Build history of the part. All positions in model axes, mm. Coordinates: 2 decimals unless noted, no trailing zeros. Loops run counter-clockwise (first coordinate to the right, second up) from the corner with the lowest first, then second, coordinate; pieces in that order, holes last. Notation, with made-up numbers: (-0.75, 59.25) - (33.25, 59.25) arc R25 ccw to (33.25, 88.25) - close; hole circle Ø10 at (59, -22). An arc over 180 degrees is marked (long way). One line per item, written item: value.
```python
from build123d import *

# Parameters (mm, degrees)
BOSS_EXTRUDE1_DEPTH                          = 2.5
CSK_FOR_M2_5_COUNTERSUNK_FLAT_HEAD_S_2_COUNT = 2
CSK_FOR_M2_5_COUNTERSUNK_FLAT_HEAD_S_2_PITCH = 24
CSK_FOR_M2_5_COUNTERSUNK_FLAT_HEAD_S_3_COUNT = 2
CSK_FOR_M2_5_COUNTERSUNK_FLAT_HEAD_S_3_PITCH = 114
CSK_FOR_M2_5_COUNTERSUNK_FLAT_HEAD_S_4_COUNT = 2
CSK_FOR_M2_5_COUNTERSUNK_FLAT_HEAD_S_4_PITCH = 116.498927034
SKETCH4_R                                    = 10.25
CUT_EXTRUDE1_DEPTH                           = 132.231695022


with BuildPart() as part:
    # Sketch1 → Boss-Extrude1 (new body)
    with BuildSketch(Plane.XY):
        with BuildLine():
            Line((-63.122572744, 90.432106023), (-63.122572744, -25.567893977))
            ThreePointArc((-63.122572744, -25.567893977), (-63.708359182, -26.98210754), (-65.122572744, -27.567893977))
            Line((-65.122572744, -27.567893977), (-91.122572744, -27.567893977))
            ThreePointArc((-91.122572744, -27.567893977), (-92.536786306, -26.98210754), (-93.122572744, -25.567893977))
            Line((-93.122572744, -25.567893977), (-93.122572744, 90.432106023))
            ThreePointArc((-93.122572744, 90.432106023), (-92.536786306, 91.846319585), (-91.122572744, 92.432106023))
            Line((-91.122572744, 92.432106023), (-65.122572744, 92.432106023))
            ThreePointArc((-65.122572744, 92.432106023), (-63.708359182, 91.846319585), (-63.122572744, 90.432106023))
        make_face()
    extrude(amount=BOSS_EXTRUDE1_DEPTH)

    # Sketch3 → CSK for M2.5 Countersunk Flat Head Screw2 (revolve, cut)
    with BuildSketch(Plane(origin=(-66.122572744, 89.432106023, 0), x_dir=(0, 1, 0), z_dir=(1, 0, 0))):
        Polygon((0, 0), (0, 2.5), (1.45, 2.5), (1.45, 1.3), (2.75, 0), align=None)
    csk_for_m2_5_countersunk_flat_head_screw = revolve(axis=Axis((-66.122572744, 89.432106023, -6.35), (0, 0, 1)), mode=Mode.SUBTRACT)

    # CSK for M2.5 Countersunk Flat Head S 2: CSK for M2.5 Countersunk Flat Head Screw2 ×2
    with Locations(*[(-i * CSK_FOR_M2_5_COUNTERSUNK_FLAT_HEAD_S_2_PITCH, 0, 0) for i in range(1, CSK_FOR_M2_5_COUNTERSUNK_FLAT_HEAD_S_2_COUNT)]):
        add(csk_for_m2_5_countersunk_flat_head_screw, mode=Mode.SUBTRACT)

    # CSK for M2.5 Countersunk Flat Head S 3: CSK for M2.5 Countersunk Flat Head Screw2 ×2
    with Locations(*[(0, -i * CSK_FOR_M2_5_COUNTERSUNK_FLAT_HEAD_S_3_PITCH, 0) for i in range(1, CSK_FOR_M2_5_COUNTERSUNK_FLAT_HEAD_S_3_COUNT)]):
        add(csk_for_m2_5_countersunk_flat_head_screw, mode=Mode.SUBTRACT)

    # CSK for M2.5 Countersunk Flat Head S 4: CSK for M2.5 Countersunk Flat Head Screw2 ×2
    with Locations(*[Vector(-0.20601048104984201, -0.978549784986749, 0) * (i * CSK_FOR_M2_5_COUNTERSUNK_FLAT_HEAD_S_4_PITCH) for i in range(1, CSK_FOR_M2_5_COUNTERSUNK_FLAT_HEAD_S_4_COUNT)]):
        add(csk_for_m2_5_countersunk_flat_head_screw, mode=Mode.SUBTRACT)

    # Sketch4 → Cut-Extrude1 (cut, through all)
    with BuildSketch(Plane(origin=(0, 0, 0), x_dir=(-1, 0, 0), z_dir=(0, 0, -1))):
        with Locations((76.682572744, 32.432106023)):
            Circle(SKETCH4_R)
    extrude(amount=-CUT_EXTRUDE1_DEPTH, mode=Mode.SUBTRACT)


solid = part.part
```
Item 1: Cut at A-A, the plane x = -83.25. Write the cut outline in (y, z).
Check result:
outline: (-27.57, 0) - (24.56, 0) - (24.56, 2.5) - (-27.57, 2.5) - close; (40.3, 0) - (92.43, 0) - (92.43, 2.5) - (40.3, 2.5) - close
Item 2: Probe probe 1 along Y at (x, z) = (-76.5, 1); probe 2 along X at (y, z) = (35, 1.75); probe 3 along Y at (x, z) = (-66, 0.95). List the from-to ranges inside material, lowest first. Write a range as from..to.
Check result:
probe 1: y = -27.57..22.18, 42.68..92.43
probe 2: x = -93.12..-86.61, -66.76..-63.12
probe 3: y = -27.57..-26.36, -22.77..87.64, 91.23..92.43
Item 3: Pull direction X, two halves, no side cores. Call faces 1 (the face through (-91.345, 90.212, 1.892)), 2 (the face through (-78, -27.568, 1)), 3 (the face through (-63.72, 91.86, 1.23)): released by +X, released by -X, zero draft, split by the parting line, or undercut.
Check result:
face 1: undercut
face 2: zero draft
face 3: released by +X
Item 4: Cut at B-B, the plane y = 27.5. Write the cut outline in (x, z), then the cut area to 3 significant figures.
Check result:
outline: (-93.12, 0) - (-85.67, 0) - (-85.67, 2.5) - (-93.12, 2.5) - close; (-67.7, 0) - (-63.12, 0) - (-63.12, 2.5) - (-67.7, 2.5) - close
area: 30.1 mm^2
Item 5: Drop flat-ended pins along their axis: P1, Ø2.5, axis at x = -66.12, y = 89.43, coming from the -Z side; P2, Ø4, axis at x = -90.12, y = -24.57, coming from the -Z side. Give the stop position or say it passes through.
Check result:
P1: passes through
P2: stops at z = 0.75
